```python
from build123d import *

# Parameters (mm, degrees)
F0_W           = 25
F0_H           = 30
F1_DEPTH       = 4
F2_W           = 25
F2_H           = 11
F3_DEPTH       = 13
F4_R           = 1.675
F5_DEPTH       = 25
F5_DEPTH_BACK  = 25
F7_DEPTH       = 6
F8_R           = 8
F9_DEPTH       = 6
F4_R_2         = 3
F10_DEPTH      = 2
F10_DEPTH_BACK = 25
F12_DEPTH      = 2
F13_W          = 11
F13_H          = 17
F14_DEPTH      = 2
F15_R          = 1.45
F16_DEPTH      = 25
F17_T1_DEPTH   = 42
F17_T6_DEPTH   = 41.9721204096
F17_T11_DEPTH  = 41.9721204096
F18_DEPTH      = 9
F19_DEPTH      = 13
F21_DEPTH      = 28


# Not quite as in the source:
# - a fillet or chamfer that OpenCascade refuses, or shapes differently, is made with other operations: its cross-section is extruded or revolved along the edge and cut away or added
# - a feature names something its author has since deleted; it is built from what else it names


with BuildPart() as f1:
    # F0 (on Top) → F1 (new body)
    with BuildSketch(Plane.XY):
        with Locations((12.5, 15)):
            Rectangle(F0_W, F0_H)
    extrude(amount=F1_DEPTH)

    # F2 (on face) → F3 (join)
    with BuildSketch(Plane.XY.offset(4)):
        with Locations((12.5, 24.5)):
            Rectangle(F2_W, F2_H)
    extrude(amount=F3_DEPTH)

    # F4 (on face) → F5 (cut, two sides)
    with BuildSketch(Plane.XY.offset(4)) as f5_sk:
        with Locations((5, 21)):
            Circle(F4_R)
        with Locations((20, 21)):
            Circle(F4_R)
        with Locations((20, 6)):
            Circle(F4_R)
        with Locations((5, 6)):
            Circle(F4_R)
    extrude(amount=-F5_DEPTH, mode=Mode.SUBTRACT)
    extrude(f5_sk.sketch, amount=F5_DEPTH_BACK, mode=Mode.SUBTRACT)

    # F6 (on face) → F7 (cut)
    with BuildSketch(Plane(origin=(0, 30, 0), x_dir=(-1, 0, 0), z_dir=(0, 1, 0))):
        with BuildLine():
            ThreePointArc((-18.5, 17), (-12.5, 11), (-6.5, 17))
            Line((-6.5, 17), (-18.5, 17))
        make_face()
    extrude(amount=-F7_DEPTH, mode=Mode.SUBTRACT)

    # F8 (on face) → F9 (cut)
    with BuildSketch(Plane.XZ.offset(-19)):
        with Locations((12.5394891948, 17)):
            Circle(F8_R)
    extrude(amount=-F9_DEPTH, mode=Mode.SUBTRACT)

    # F4 (on face) → F10 (cut, two sides)
    with BuildSketch(Plane.XY.offset(4)) as f10_sk:
        with BuildLine():
            ThreePointArc((7.2360679775, 19), (7.8025170769, 19.9295337307), (8, 21))
            ThreePointArc((8, 21), (3.9295337307, 23.8025170769), (2.7639320225, 19))
            Line((2.7639320225, 19), (7.2360679775, 19))
        make_face()
        with Locations((5, 21)):
            Circle(F4_R, mode=Mode.SUBTRACT)
        with BuildLine():
            ThreePointArc((23, 21), (18.9295337307, 23.8025170769), (17.7639320225, 19))
            Line((17.7639320225, 19), (22.2360679775, 19))
            ThreePointArc((22.2360679775, 19), (22.8025170769, 19.9295337307), (23, 21))
        make_face()
        with Locations((20, 21)):
            Circle(F4_R, mode=Mode.SUBTRACT)
        with Locations((20, 6)):
            Circle(F4_R_2)
        with Locations((20, 6)):
            Circle(F4_R, mode=Mode.SUBTRACT)
        with Locations((5, 6)):
            Circle(F4_R_2)
        with Locations((5, 6)):
            Circle(F4_R, mode=Mode.SUBTRACT)
        with BuildLine():
            Line((22.2360679775, 19), (17.7639320225, 19))
            ThreePointArc((17.7639320225, 19), (20, 18), (22.2360679775, 19))
        make_face()
        with BuildLine():
            Line((7.2360679775, 19), (2.7639320225, 19))
            ThreePointArc((2.7639320225, 19), (5, 18), (7.2360679775, 19))
        make_face()
    extrude(amount=-F10_DEPTH, mode=Mode.SUBTRACT)
    extrude(f10_sk.sketch, amount=F10_DEPTH_BACK, mode=Mode.SUBTRACT)

    # F11 (on face) → F12 (join)
    with BuildSketch(Plane(origin=(0, 0, 0), x_dir=(0, -1, 0), z_dir=(-1, 0, 0))):
        Polygon((-30, 17), (-30, 0), (-19, 0), (-19, 4), (-19, 17), align=None)
    extrude(amount=F12_DEPTH)

    # F13 (on face) → F14 (join)
    with BuildSketch(Plane.YZ.offset(25)):
        with Locations((24.5, 8.5)):
            Rectangle(F13_W, F13_H)
    extrude(amount=F14_DEPTH)

    # F15 (on face) → F16 (cut)
    with BuildSketch(Plane.XY.offset(17)):
        with Locations((0.45, 25.55)):
            Circle(F15_R)
        with Locations((24.55, 25.55)):
            Circle(F15_R)
    extrude(amount=-F16_DEPTH, mode=Mode.SUBTRACT)

    # F17: fillet of radius 5 on 4 edges, made by hand

    # F17_s2 → F17_t1 (cut)
    with BuildSketch(Plane.XY.offset(-12.5)):
        with BuildLine():
            ThreePointArc((-2, 25), (-0.5355339059, 28.5355339059), (3, 30))
            Line((3, 30), (-2, 30))
            Line((-2, 30), (-2, 25))
        make_face()
        with BuildLine():
            ThreePointArc((22, 30), (25.5355339059, 28.5355339059), (27, 25))
            Line((27, 25), (27, 30))
            Line((27, 30), (22, 30))
        make_face()
    extrude(amount=F17_T1_DEPTH, mode=Mode.SUBTRACT)


with BuildPart() as f17_tool4:
    # F17_s5 → F17_t6 (new body)
    with BuildSketch(Plane.XY.offset(29.4860602048)):
        with BuildLine():
            ThreePointArc((2.7639320225, 19), (-0.6180339887, 20.5433619184), (-2, 23.9944240819))
            Line((-2, 23.9944240819), (-2, 19))
            Line((-2, 19), (2.7639320225, 19))
        make_face()
    extrude(amount=-F17_T6_DEPTH)

    split(bisect_by=Plane.YZ, keep=Keep.BOTTOM)


with BuildPart() as f1_1:
    add(f1.part)

    # F17_t3: cut F17_tool4
    add(f17_tool4.part, mode=Mode.SUBTRACT)


with BuildPart() as f17_tool9:
    # F17_s10 → F17_t11 (new body)
    with BuildSketch(Plane.XY.offset(29.4860602048)):
        with BuildLine():
            ThreePointArc((22.2360679775, 19), (25.6180339887, 20.5433619184), (27, 23.9944240819))
            Line((27, 23.9944240819), (27, 19))
            Line((27, 19), (22.2360679775, 19))
        make_face()
    extrude(amount=-F17_T11_DEPTH)

    split(bisect_by=Plane.YZ.offset(25), keep=Keep.TOP)


with BuildPart() as f1_2:
    add(f1_1.part)

    # F17_t8: cut F17_tool9
    add(f17_tool9.part, mode=Mode.SUBTRACT)

    # F18 (add): a face of the model
    f18_faces = [f1_2.faces().sort_by_distance(p)[0] for p in [
        (12.5, 0, 2),
    ]]
    extrude(f18_faces, amount=F18_DEPTH)

    # F19 (add): a face of the model
    f19_faces = [f1_2.faces().sort_by_distance(p)[0] for p in [
        (12.5, 4.7791140559, 4),
    ]]
    extrude(f19_faces, amount=F19_DEPTH)

    # F20 (on face) → F21 (cut, through all)
    with BuildSketch(Plane.XZ.offset(9)):
        with BuildLine():
            ThreePointArc((1, 17), (12.5, 5.5), (24, 17))
            Line((24, 17), (1, 17))
        make_face()
    extrude(amount=-F21_DEPTH, mode=Mode.SUBTRACT)


solid = f1_2.part
```
The model under review builds one solid part; all positions refer to its coordinate system, in mm. A direction names the side the tool comes from. Round coordinates to 2 decimals unless told otherwise and drop trailing zeros. Write each loop counter-clockwise with the first axis right and the second up, starting at its lowest first coordinate (ties: lowest second). Pieces come first, ordered by that corner, then holes. Notation, with made-up numbers: (82.5, 39.5) - (134.5, 39.5) arc R13 cw to (134.5, 48.5) - close; hole circle Ø6 at (56.5, 29.5). An arc over 180 degrees is marked (long way). Answer as CSV lines item,"result". Start each with the question number.
(1) We need section A-A on z = 16.25. State the section outline as (x, y) points.
(2) We need section C-C on x = 5.25. State the section outline as (y, z) points, plus the area to 3 significant figures.
(3) We need section B-B on x = 24.55. State the section outline as (y, z) points, plus the area to 3 significant figures.
(4) Draft analysis for pull direction X (two halves, no side actions). For faces 1 (the flat face through (27, 24.5, 8.6)), 2 (the flat face through (6.3, 4.7, 2)), 3 (the flat face through (12, 30, 6)), 4 (the cylindrical face through (-1, 28, 8)), state which applies: pulls with the +X half, pulls with the -X half, needs draft (parallel to the pull), parting line crosses it, or undercut.
(5) For faces 5 (the cylindrical face through (0.136, 24.134, 8.619)), 6 (the flat face through (25, 5, 8)), 7 (the cylindrical face through (-1.46, 21.73, 8.62)), 8 (the flat face through (21.3, 4.7, 2)), 9 (the flat face through (2, 19, 15)), list the 3-axis set-ups (+Z, -Z, +X, -X, +Y, -Y) from which the entire face can be reached by the end or side of a thin tool; tool diameter is ignored.
(6) We need section D-D on y = 25.55. State the section outline as (x, z) points.
(7) For pin 1 Ø4 at (x, y) = (12, 15.5) entering from +Z (3 decimals); pin 2 Ø1.5 at (y, z) = (15.5, 5) entering from -X; pin 3 Ø4 at (x, y) = (5, 6) entering from +Z; pin 4 Ø2.5 at (x, y) = (24.55, 25.55) entering from -Z, all flat-tipped, find the tip position at first contact; note any pin that passes through.
(8) To check wall thickness, follow line 1 (Y direction, x = 20, z = 0.8) (3 decimals); line 2 (Y direction, x = 5, z = 2.95); line 3 (Y direction, x = 14, z = 9.5). State the ranges of each line that lie inside material, in increasing order.
Worked answers:
1,outline,"(-2, 23.99) arc R5 ccw to (0, 19.99) - (0, -9) - (1.02, -9) - (1.02, 19) - (2.76, 19) arc R3 cw to (4.57, 23.97) - (4.57, 25) - (6.55, 25) - (6.55, 30) - (3, 30) arc R5 ccw to (-2, 25) - close; (18.45, 25) - (20.5, 25) - (20.5, 23.96) arc R3 cw to (22.24, 19) - (23.98, 19) - (23.98, -9) - (25, -9) - (25, 19.99) arc R5 ccw to (27, 23.99) - (27, 25) arc R5 ccw to (22, 30) - (18.45, 30) - close; hole circle Ø2.9 at (0.45, 25.55); hole circle Ø2.9 at (24.55, 25.55)"
2,outline,"(-9, 0) - (4.34, 0) - (4.34, 2) - (3.01, 2) - (3.01, 8.07) - (-9, 8.07) - close; (7.66, 0) - (19.34, 0) - (19.34, 2) - (18.01, 2) - (18.01, 8.07) - (8.99, 8.07) - (8.99, 2) - (7.66, 2) - close; (22.66, 0) - (30, 0) - (30, 17) - (25, 17) - (25, 13.7) - (23.99, 13.7) - (23.99, 2) - (22.66, 2) - close"
2,area,"279 mm²"
3,outline,"(-9, 0) - (24.1, 0) - (24.1, 17) - (-9, 17) - close; (27, 0) - (29.3, 0) - (29.3, 17) - (27, 17) - close"
3,area,"602 mm²"
4,face 1,"pulls with the +X half"
4,face 2,"undercut"
4,face 3,"needs draft"
4,face 4,"pulls with the -X half"
5,face 5,"+Z, -Z"
5,face 6,"+Z, -Z, +X, -Y"
5,face 7,"+Z, -Z, -X, -Y"
5,face 8,"+Z"
5,face 9,"+Z, -Y"
6,outline,"(-1.97, 0) - (-1, 0) - (-1, 17) - (-1.97, 17) - close; (1.9, 0) - (23.1, 0) - (23.1, 17) - (18.5, 17) arc R6 cw to (6.5, 17) - (1.9, 17) - close; (26, 0) - (26.97, 0) - (26.97, 17) - (26, 17) - close"
7,pin 1,"z = 5.775"
7,pin 2,"x = 0"
7,pin 3,"z = 2"
7,pin 4,"through"
8,line 1,"-9 to 4.325, 7.675 to 19.325, 22.675 to 30"
8,line 2,"-9 to 3, 9 to 18, 24 to 30"
8,line 3,"25 to 30"
